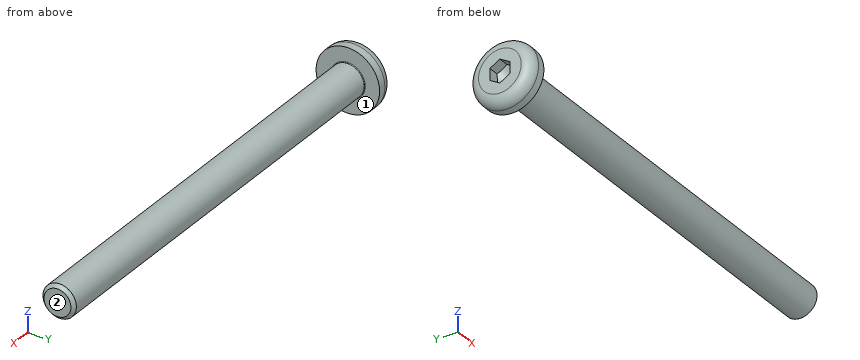
Autodesk Inventor part; units mm, degrees
ref_plane "Work Plane1" through (29, 0, 0) normal (0, -1, 0) x (1, 0, 0)
ref_plane "YZ Plane" through (0, 0, 0) normal (1, 0, 0) x (0, 1, 0)
ref_plane "XZ Plane" through (0, 0, 0) normal (0, 1, 0) x (-1, 0, 0)
sketch "Sketch1" plane through (0, 0, 0) normal (0, 0, 1) x (1, 0, 0)
  line L0 (-0.19, 0) -> (65, 0)
  line L1 (65, 0) -> (65, 2.5)
  line L2 (65, 2.5) -> (2, 2.5)
  line L3 (2, 2.5) -> (1.5091, 2.5)
  line L4 (1.5091, 2.5) -> (0, 2.5)
  line L5 (0, 2.5) -> (0, 4.75)
  line L6 (0, 4.75) -> (-2.75, 4.75)
  line L7 (-2.75, 4.75) -> (-2.75, 1.7321)
  line L8 (-2.75, 1.7321) -> (-1.19, 1.7321)
  line L9 (-1.19, 1.7321) -> (-0.19, 0)
  line L10 (-16.3, 0) -> (78.55, 0)
  line L11 (0, -0.95) -> (0, 5.7)
  line L12 (2, 2.5) -> (0, 2.5) construction
  dimension "d1" = 63
  dimension "d2" = 0.4909
  dimension "d3" = 2.75
  dimension "d4" = 1.56
  dimension "d5" = 60
  dimension "d6" = 5
  dimension "d7" = 5
  dimension "d8" = 3.4641
  dimension "d9" = 9.5
  dimension "d26" = 65
revolve "Body" add sketch "Sketch1" angle 360 about axis through (-0.19, 0, 0) along (1, 0, 0)
sketch "Sketch2" plane through (-2.75, 0, 0) normal (-1, 0, 0) x (0, 0, 1)
  circle A0 centre (0, 0) radius 1.7321
  line L0 (0, -6.65) -> (0, 6.65)
  line L1 (-6.65, 0) -> (6.65, 0)
  line L2 (1.7321, 0) -> (0.866, -1.5)
  line L3 (0.866, -1.5) -> (-0.866, -1.5)
  line L4 (-0.866, -1.5) -> (-1.7321, 0)
  line L5 (-1.7321, 0) -> (-0.866, 1.5)
  line L6 (-0.866, 1.5) -> (0.866, 1.5)
  line L7 (0.866, 1.5) -> (1.7321, 0)
extrude "Slot" add sketch "Sketch2" against normal up to next contours L7 A0 | A0 L2 | L6 L0 A0 | A0 L0 L3 | L0 L6 A0 | A0 L3 L0 | L4 A0 | A0 L5
fillet "Fillet1" radius 1.56 1 edges at (-2.75, -4.75, 0)
thread "Thread"
chamfer "Chamfer1" distance 0.4908 distance2 0.4908 1 edges at (65, -2.5, 0) measured on face at (65, 0.695, -0.3648)
ref_plane "Work Plane1" through (29, 0, 0) normal (0, -1, 0) x (1, 0, 0)
fillet "Fillet2" radius 0.1 1 edges at (0, -2.5, 0)
equation "\"d1\" = GEL"
equation "\"d3\" = KOH"
equation "\"d4\" = INTI"
equation "\"d6\" = GD"
equation "\"d7\" = BDM"
equation "\"d8\" = 1.1547 * SW"
equation "\"d9\" = KOD"
equation "\"d26\" = NLG"
equation "\"d30\" = R"
equation "\"d17\" = RR"
equation "\"d13\" = GEL"
equation "\"d15\" = -0.5 * SPD + 0.5 * GD"
equation "\"d16\" = GUL"
equation "\"GD\" = NND"
equation "\"NLG\" = 65"
equation "\"GEL\" = 63"
equation "\"KOD\" = 9.5"
equation "\"KOH\" = 2.75"
equation "\"INTI\" = 1.56"
equation "\"GAL\" = 0.61345 * PTC"
equation "\"GUL\" = 0.61345 * PTC"
equation "\"BDM\" = NND"
equation "\"SW\" = 3"
equation "\"RR\" = INTI"
equation "\"SPD\" = NND - 1.2269 * PTC"
equation "\"R\" = 0.1"
equation "\"KR\" = 5.2"
equation "\"GD1\" = THREADDIA - 1.2269 * PTC"
equation "\"THREADDIA\" = 5"
equation "\"FAWI\" = 45deg"
equation "\"PTC\" = 0.8"
equation "\"KOH1\" = 1.56"
equation "\"NND\" = 5"
equation "\"TOA\" = 30deg"
equation "\"E0\" = 1.155 * SW"
properties part number "Unbrako - M5 x 65" material "Steel, Mild"
Part model, mm, in its own coordinate system. Face numbers are marked on the shaded views. A direction names the side the tool comes from. Give positions to 0.01 mm unless a question says otherwise; leave off trailing zeros. Loops run counter-clockwise (first coordinate to the right, second up) from the corner with the lowest first, then second, coordinate; pieces in that order, holes last.
(1) Drill centre lines: line 1 along X through (y, z) = (2.75, 1); line 2 along Y through (x, z) = (26.5, -0.25). Where is each one in solid material? Low to high.
Return value:
line 1: x = -2.75 to 0
line 2: y = -2.49 to 2.49
(2) Band-saw the part on A-A (x = 18). Write the cut outline in (y, z), and give its area (3 significant figures).
Return value:
outline: circle Ø5 at (0, 0)
area: 19.6 mm2
(3) Pin check, flat tips, straight feed: pin 1 (4 mm diameter, centred on x = 12, z = 3.5, fed in from +Y); pin 2 (0.5 mm diameter, centred on x = -2.5, z = 0, fed in from +Y); pin 3 (1 mm diameter, centred on x = 24.5, y = -4, fed in from +Z); pin 4 (4 mm diameter, centred on x = 34, z = -3, fed in from +Y). Stop position of each tip, or through.
Return value:
pin 1: stops at y = 2
pin 2: stops at y = 4.33
pin 3: passes through
pin 4: stops at y = 2.29
(4) 3-axis set-ups, long thin cutter, end or side, ignore diameter. For the marked faces 1 and 2: which of +Z, -Z, +X, -X, +Y, -Y reach the whole face in a straight line?
Return value:
face 1: +X
face 2: +Z, -Z, +X, +Y, -Y
